```python
from build123d import *

# Parameters (mm, degrees)
F0_W            = 152.4
F0_H            = 152.4
F1_DEPTH        = 60.325
F2_DEPTH        = 49.2125
F2_COPIES_COUNT = 4
F3_DEPTH        = 11.1125
F3_COPIES_COUNT = 4
F0_R            = 317.5
F4_DEPTH        = 49.2125


# Not quite as in the source:
# - a pattern or mirror of a feature is missing from the dataset's text; its kind, count and spacing are read off the source's solid


with BuildPart() as f1:
    # F0 (on Right) → F1 (new body, symmetric)
    with BuildSketch(Plane.YZ):
        Polygon((101.6, -101.6), (101.6, 65.6789755157), (101.6, 92.6197438789), (101.6, 101.6), (92.6197438789, 101.6), (65.6789755157, 101.6), (-101.6, 101.6), (-101.6, -101.6), align=None)
        Rectangle(F0_W, F0_H, mode=Mode.SUBTRACT)
    extrude(amount=F1_DEPTH, both=True)

    # F0 (on Right) → F2 (join, symmetric)
    with BuildSketch(Plane.YZ):
        with BuildLine():
            Line((101.6, 92.6197438789), (219.9694977227, 210.9892416016))
            ThreePointArc((219.9694977227, 210.9892416016), (215.5261469057, 215.5261469057), (210.9892416016, 219.9694977227))
            Line((210.9892416016, 219.9694977227), (92.6197438789, 101.6))
            Line((92.6197438789, 101.6), (101.6, 101.6))
            Line((101.6, 101.6), (101.6, 92.6197438789))
        make_face()
    f2 = extrude(amount=F2_DEPTH, both=True)

    # F2_copies: F2 ×4 about axis
    f2_copies_axis = Axis((0, 0, 0), (1, 0, 0))
    for i in range(1, F2_COPIES_COUNT):
        add(f2.rotate(f2_copies_axis, i * 360 / F2_COPIES_COUNT))

    # F0 (on Right) → F3 (join, symmetric)
    with BuildSketch(Plane.YZ):
        with BuildLine():
            ThreePointArc((210.9892416016, 219.9694977227), (204.0025151944, 226.4641556502), (196.815976229, 232.7370007133))
            Line((196.815976229, 232.7370007133), (65.6789755157, 101.6))
            Line((65.6789755157, 101.6), (92.6197438789, 101.6))
            Line((92.6197438789, 101.6), (210.9892416016, 219.9694977227))
        make_face()
        with BuildLine():
            Line((101.6, 65.6789755157), (232.7370007133, 196.815976229))
            ThreePointArc((232.7370007133, 196.815976229), (226.4641556502, 204.0025151944), (219.9694977227, 210.9892416016))
            Line((219.9694977227, 210.9892416016), (101.6, 92.6197438789))
            Line((101.6, 92.6197438789), (101.6, 65.6789755157))
        make_face()
    f3 = extrude(amount=F3_DEPTH, both=True)

    # F3_copies: F3 ×4 about axis
    f3_copies_axis = Axis((0, 0, 0), (1, 0, 0))
    for i in range(1, F3_COPIES_COUNT):
        add(f3.rotate(f3_copies_axis, i * 360 / F3_COPIES_COUNT))

    # F0 (on Right) → F4 (join, symmetric)
    with BuildSketch(Plane.YZ):
        Circle(F0_R)
        with BuildLine():
            ThreePointArc((232.7370007133, 196.815976229), (286.2178172454, 104.7969517271), (304.8, 0))
            ThreePointArc((304.8, 0), (-276.4891946845, -128.2839242567), (196.815976229, 232.7370007133))
            ThreePointArc((196.815976229, 232.7370007133), (204.0025151944, 226.4641556502), (210.9892416016, 219.9694977227))
            ThreePointArc((210.9892416016, 219.9694977227), (215.5261469057, 215.5261469057), (219.9694977227, 210.9892416016))
            ThreePointArc((219.9694977227, 210.9892416016), (226.4641556502, 204.0025151944), (232.7370007133, 196.815976229))
        make_face(mode=Mode.SUBTRACT)
    extrude(amount=F4_DEPTH, both=True)


solid = f1.part
```
Geometry: final body of the model. Coordinates: model frame, mm. A direction names the side the tool comes from. Round coordinates to 2 decimals unless told otherwise and drop trailing zeros. Order: outer loops, then holes, each group sorted by start corner. A loop starts at its lowest first (then second) coordinate and runs counter-clockwise, first axis right, second up. Notation, with made-up numbers: (22.5, 78.5) -> (55.5, 78.5) arc R14 ccw to (55.5, 84.5) -> close; hole circle Ø6 at (-13.5, -17.5). An arc over 180 degrees is marked (long way). Use CSV: the item, a comma, the result in double quotes. Start each with the question number.
1) Section D-D (y = -255). Return the cut outline in (x, z), and give its area (3 significant figures).
2) Draft query along Y for faces 1 (the face through (0.69, 302.84, 95.37)), 2 (the face through (-49.212, -119, 119)), 3 (the face through (0.689, -304.783, -3.262)). Return one class per face: +Y half, -Y half, draft (parallel to the pull), parting line (faces both ways), or undercut.
3) Section A-A (y = 0). Return the cut outline in (x, z) (1 decimal), and give its area (3 significant figures).
4) Section C-C (z = -247.5). Return the cut outline in (x, y).
5) Set-up query: faces 4 (the face through (1, -101.6, 1)), 5 (the face through (30.43, -152.63, -161.61)), 6 (the face through (1, 76.2, -1)). Return all of +Z, -Z, +X, -X, +Y, -Y with unobstructed straight access to the full face (end or side cutting, diameter ignored); none if empty.
6) Material intervals for line 1 along Y through (x, z) = (10, 9); line 2 along Y through (x, z) = (18, -4); line 3 along Z through (x, y) = (-3, 159.5), sorted ascending. Write a range as from..to.
7) First-contact query: pin 1 Ø1 at (x, y) = (16.5, -114) entering from +Z; pin 2 Ø6 at (x, z) = (35.5, 190) entering from -Y; pin 3 Ø8 at (y, z) = (-136.5, -170) entering from +X. Flat tips, straight axial feed; report the tip coordinate or a pass-through.
Returned:
1,outline,"(-49.21, -189.16) -> (49.21, -189.16) -> (49.21, -166.97) -> (-49.21, -166.97) -> close; (-49.21, 166.97) -> (49.21, 166.97) -> (49.21, 189.16) -> (-49.21, 189.16) -> close"
1,area,"4,370 mm²"
2,face 1,"parting line"
2,face 2,"draft"
2,face 3,"undercut"
3,outline,"(-60.3, -101.6) -> (60.3, -101.6) -> (60.3, -76.2) -> (-60.3, -76.2) -> close; (-60.3, 76.2) -> (60.3, 76.2) -> (60.3, 101.6) -> (-60.3, 101.6) -> close; (-49.2, -317.5) -> (49.2, -317.5) -> (49.2, -304.8) -> (-49.2, -304.8) -> close; (-49.2, 304.8) -> (49.2, 304.8) -> (49.2, 317.5) -> (-49.2, 317.5) -> close"
3,area,"8,630 mm²"
4,outline,"(-49.21, -198.87) -> (49.21, -198.87) -> (49.21, -177.9) -> (-49.21, -177.9) -> close; (-49.21, 177.9) -> (49.21, 177.9) -> (49.21, 198.87) -> (-49.21, 198.87) -> close"
5,face 4,"none"
5,face 5,"+X"
5,face 6,"+X, -X"
6,line 1,"y = -317.37..-304.67, -101.6..-76.2, 76.2..101.6, 304.67..317.37"
6,line 2,"y = -317.47..-304.77, -101.6..-76.2, 76.2..101.6, 304.77..317.47"
6,line 3,"z = -274.53..-259.74, -195.42..-123.58, 123.58..195.42, 259.74..274.53"
7,pin 1,"stops at z = 296.52"
7,pin 2,"stops at y = -256.59"
7,pin 3,"stops at x = 11.11"
